Here's how the part is built. I have some questions about the finished solid (model axes, mm). A direction names the side the tool comes from. Give positions to 0.01 mm unless a question says otherwise; leave off trailing zeros. Loops run counter-clockwise (first coordinate to the right, second up) from the corner with the lowest first, then second, coordinate; pieces in that order, holes last.
Q1. I need wall thicknesses on probe 1 along X at (y, z) = (-6.75, 6); probe 2 along Z at (x, y) = (47, -6); probe 3 along Y at (x, z) = (27.5, 9.5). Which ranges of each line are inside material? Lowest first, please.
Q2. For faces 5 (the face through (20, -10, 6)), 6 (the face through (44.1, 0, 4.6)), 7 (the face through (-10.9, 0, 4.6)), which set-ups out of +Z, -Z, +X, -X, +Y, -Y let a thin tool reach every point of the face, with its end or its side?
Q3. Suppose I cut it at A-A (z = 6). List the corners of the cut face in (x, y) for me.
Q4. Suppose I cut it at C-C (x = 16). List the corners of the cut face in (y, z) for me.
Q5. Suppose I cut it at D-D (z = 11). List the corners of the cut face in (x, y) for me, and give its area (3 significant figures).
Q6. Thinking about a two-plate mould opening in Z: for faces 1 (the face through (51, -5, 6)), 2 (the face through (20, 18, 12)), 3 (the face through (40, 25, 6)), 4 (the face through (20, 18, 0)), which applies, pulls with the +Z half, pulls with the -Z half, needs draft (parallel to the pull), parting line crosses it, or undercut?
Q7. Suppose I cut it at B-B (y = -4.5). List the corners of the cut face in (x, z) for me.
Q8. I'm going to push flat-ended pins straight in: P1, Ø3.5, axis at x = -9, z = 7, coming from the +Y side; P2, Ø1, axis at x = 35, z = 10, coming from the +Y side. Where does each tip first touch, or does it pass through?
```python
from build123d import *

# Parameters (mm, degrees)
SKETCH_1_R          = 13.15
EXTRUDE_1_DEPTH     = 12
SKETCH_2_R          = 3.5
CUT_EXTRUDE_2_DEPTH = 83.273932688
SKETCH_3_R          = 3.5
CUT_EXTRUDE_3_DEPTH = 83.273932688
CHAMFER_1_SIZE      = 10
CHAMFER_2_SIZE      = 10


with BuildPart() as part:
    # 草圖1 → 填料-伸長1 (new body)
    with BuildSketch(Plane.XY):
        Polygon((40, 0), (55, 0), (55, -10), (-15, -10), (-15, 0), (0, 0), (0, 60), (40, 60), align=None)
        with Locations((20, 39)):
            Circle(SKETCH_1_R, mode=Mode.SUBTRACT)
    extrude(amount=EXTRUDE_1_DEPTH)

    # 草圖2 → 除料-伸長2 (cut, through all)
    with BuildSketch(Plane(origin=(0, 0, 0), x_dir=(1, 0, 0), z_dir=(0, 1, 0))):
        with Locations(Location((47.5, -6, 0), (0, 0, 270))):
            Circle(SKETCH_2_R)
    extrude(amount=-CUT_EXTRUDE_2_DEPTH, mode=Mode.SUBTRACT)

    # 草圖3 → 除料-伸長3 (cut, through all)
    with BuildSketch(Plane(origin=(0, 0, 0), x_dir=(1, 0, 0), z_dir=(0, 1, 0))):
        with Locations(Location((-7.5, -6, 0), (0, 0, 270))):
            Circle(SKETCH_3_R)
    extrude(amount=-CUT_EXTRUDE_3_DEPTH, mode=Mode.SUBTRACT)

    # 導角1
    chamfer_1_edges = [part.edges().sort_by_distance(p)[0] for p in [
        (0, 60, 6),
    ]]
    chamfer(chamfer_1_edges, length=CHAMFER_1_SIZE)

    # 導角2
    chamfer_2_edges = [part.edges().sort_by_distance(p)[0] for p in [
        (40, 60, 6),
    ]]
    chamfer(chamfer_2_edges, length=CHAMFER_2_SIZE)


solid = part.part
```
Solutions:
1. probe 1: x = -15 to -11, -4 to 44, 51 to 55
1. probe 2: z = 0 to 2.54, 9.46 to 12
1. probe 3: y = -10 to 28.2, 49.8 to 60
2. face 5: +Z, -Z, +X, -X, -Y
2. face 6: +Z, -Z, +X, +Y
2. face 7: +Z, -Z, -X, +Y
3. outline: (-15, -10) - (-11, -10) - (-11, 0) - (-15, 0) - close; (-4, -10) - (44, -10) - (44, 0) - (40, 0) - (40, 50) - (30, 60) - (10, 60) - (0, 50) - (0, 0) - (-4, 0) - close; (51, -10) - (55, -10) - (55, 0) - (51, 0) - close; hole circle Ø26.3 at (20, 39)
4. outline: (-10, 0) - (26.47, 0) - (26.47, 12) - (-10, 12) - close; (51.53, 0) - (60, 0) - (60, 12) - (51.53, 12) - close
5. outline: (-15, -10) - (55, -10) - (55, 0) - (40, 0) - (40, 50) - (30, 60) - (10, 60) - (0, 50) - (0, 0) - (-15, 0) - close; hole circle Ø26.3 at (20, 39)
5. area: 2,460 mm2
6. face 1: undercut
6. face 2: pulls with the +Z half
6. face 3: needs draft
6. face 4: pulls with the -Z half
7. outline: (-15, 0) - (55, 0) - (55, 12) - (-15, 12) - close; hole circle Ø7 at (-7.5, 6); hole circle Ø7 at (47.5, 6)
8. P1: stops at y = 0
8. P2: stops at y = 55.5
